from build123d import *

# Parameters (mm, degrees)
SKETCH1_R           = 3
BOSS_EXTRUDE1_DEPTH = 3.2
SKETCH1_3_R         = 1.6
BOSS_EXTRUDE2_DEPTH = 1
SKETCH5_R           = 1.5
BOSS_EXTRUDE3_DEPTH = 1
SKETCH6_R           = 2
BOSS_EXTRUDE4_DEPTH = 1
SKETCH8_R           = 1.5
BOSS_EXTRUDE5_DEPTH = 3
SKETCH10_R          = 1.8
BOSS_EXTRUDE6_DEPTH = 1
SKETCH12_R          = 1.65
CUT_EXTRUDE1_DEPTH  = 1.5


with BuildPart() as part:
    # Sketch1 → Boss-Extrude1 (new body)
    with BuildSketch(Plane(origin=(0, 0, 0), x_dir=(1, 0, 0), z_dir=(0, 1, 0))):
        with Locations((-0.522013312, 0.511138034)):
            Circle(SKETCH1_R)
    extrude(amount=BOSS_EXTRUDE1_DEPTH)

    # Sketch1<3> → Boss-Extrude2 (add)
    with BuildSketch(Plane(origin=(0, 0, 0), x_dir=(1, 0, 0), z_dir=(0, 1, 0))):
        with Locations((-0.522013312, 0.511138034)):
            Circle(SKETCH1_3_R)
    extrude(amount=BOSS_EXTRUDE2_DEPTH)

    # Sketch5 → Boss-Extrude3 (add)
    with BuildSketch(Plane.XZ):
        with Locations((-0.522013312, -0.511138034)):
            Circle(SKETCH5_R)
    extrude(amount=BOSS_EXTRUDE3_DEPTH)

    # Sketch6 → Boss-Extrude4 (add)
    with BuildSketch(Plane.XZ.offset(1)):
        with Locations((-0.522013312, -0.511138034)):
            Circle(SKETCH6_R)
    extrude(amount=BOSS_EXTRUDE4_DEPTH)

    # Sketch8 → Boss-Extrude5 (add)
    with BuildSketch(Plane(origin=(0, -2, 0), x_dir=(-1, 0, 0), z_dir=(0, -1, 0))):
        with Locations((0.522013312, 0.511138034)):
            Circle(SKETCH8_R)
    extrude(amount=BOSS_EXTRUDE5_DEPTH)

    # Sketch10 → Boss-Extrude6 (add)
    with BuildSketch(Plane.XZ.offset(5)):
        with Locations((-0.522013312, -0.511138034)):
            Circle(SKETCH10_R)
    extrude(amount=-BOSS_EXTRUDE6_DEPTH)

    # Sketch12 → Cut-Extrude1 (cut)
    with BuildSketch(Plane(origin=(0, 3.2, 0), x_dir=(1, 0, 0), z_dir=(0, 1, 0))):
        with Locations((-0.522013312, 0.511138034)):
            Circle(SKETCH12_R)
    extrude(amount=-CUT_EXTRUDE1_DEPTH, mode=Mode.SUBTRACT)


solid = part.part
Geometry check sheet. Reference: the model listing, model coordinates, mm. A direction names the side the tool comes from. Round coordinates to 2 decimals unless told otherwise and drop trailing zeros. Order: outer loops, then holes, each group sorted by start corner. A loop starts at its lowest first (then second) coordinate and runs counter-clockwise, first axis right, second up. Notation, with made-up numbers: M 38.25,27.25 L 42.25,27.25 A10 cw 42.25,42.25 Z; hole C -14.75,46.5 d6. An arc over 180 degrees is marked long. Answer in a Markdown table with one row per item. Add a question column.
Item 1: Draft check along X on faces 1 (the face through (1, 3.2, 1)), 2 (the face through (-1, 1.7, -1)), 3 (the face through (1.325, -1.493, -1.277)). Enter one of: released by +X, released by -X, zero draft, split by the parting line, or undercut.
Item 2: Sectioned sample at A-A, the plane x = -1.75. Enter the section's corners in (y, z), plus the area to 3 significant figures.
Item 3: Sectioned sample at B-B, the plane z = -1.55. Enter the section's corners in (x, y).
Item 4: Material ranges on L1, parallel to Y at x = 1.7, z = 0.4; L2, parallel to Y at x = -1.45, z = -0.5; L3, parallel to Z at x = -0.15, y = -2.5, recorded low to high. Write a range as [from, to].
Item 5: Sectioned sample at C-C, the plane y = -3.75. Enter the section's corners in (x, z), plus the area to 3 significant figures.
Item 6: Set-up check for faces 4 (the face through (-1.849, -4.507, 0.705)), 5 (the face through (-0.197, -2.986, 0.953)), 6 (the face through (1.002, 2.46, 0.121)): record each of +Z, -Z, +X, -X, +Y, -Y from which the full face is reachable in a straight line by a thin tool's end or side.
Item 7: Depth check by flat-ended pin: pin 1 Ø3 at (x, y) = (1, -0.5) entering from -Z; pin 2 Ø3 at (x, z) = (1.5, 2) entering from -Y. Enter the tip coordinate at first touch or a pass-through.
Item 8: Sectioned sample at D-D, the plane x = -3.1. Enter the section's corners in (y, z).
Filled in:
| question | item | result |
|---|---|---|
| 1 | face 1 | zero draft |
| 1 | face 2 | undercut |
| 1 | face 3 | split by the parting line |
| 2 | outline | M -5,-1.83 L -4,-1.83 L -4,-1.37 L -2,-1.37 L -2,-2.09 L -1,-2.09 L -1,-1.37 L 0,-1.37 L 0,-3.25 L 3.2,-3.25 L 3.2,-1.61 L 1.7,-1.61 L 1.7,0.59 L 3.2,0.59 L 3.2,2.23 L 0,2.23 L 0,0.35 L -1,0.35 L -1,1.07 L -2,1.07 L -2,0.35 L -4,0.35 L -4,0.8 L -5,0.8 Z |
| 2 | area | 25.2 mm² |
| 3 | outline | M -3.34,0 L -1.6,0 L -1.6,-1 L -2.23,-1 L -2.23,-2 L -1.6,-2 L -1.6,-4 L -1.99,-4 L -1.99,-5 L 0.95,-5 L 0.95,-4 L 0.56,-4 L 0.56,-2 L 1.19,-2 L 1.19,-1 L 0.56,-1 L 0.56,0 L 2.29,0 L 2.29,3.2 L 0.76,3.2 L 0.76,1.7 L -1.8,1.7 L -1.8,3.2 L -3.34,3.2 Z |
| 4 | L1 | y = [0, 3.2] |
| 4 | L2 | y = [-5, 1.7] |
| 4 | L3 | z = [-1.96, 0.94] |
| 5 | outline | C -0.52,-0.51 d3 |
| 5 | area | 7.07 mm² |
| 6 | face 4 | -Y |
| 6 | face 5 | none |
| 6 | face 6 | +Y |
| 7 | pin 1 | stops at z = -3.51 |
| 7 | pin 2 | stops at y = -5 |
| 8 | outline | M 0,-2.05 L 3.2,-2.05 L 3.2,1.02 L 0,1.02 Z |
